For this review, take the finished solid that the model builds, in its own axes (mm). A direction names the side the tool comes from. Round coordinates to 2 decimals unless told otherwise and drop trailing zeros. Write each loop counter-clockwise with the first axis right and the second up, starting at its lowest first coordinate (ties: lowest second). Pieces come first, ordered by that corner, then holes. Notation, with made-up numbers: M 74,29 L 105,29 A22 cw 105,52 Z; hole C -6.5,45.25 d7. An arc over 180 degrees is marked long. One line per question, with ' | ' between items.
```python
from build123d import *

# Parameters (mm, degrees)
F1_DEPTH = 5
F2_W     = 3
F2_H     = 7
F3_DEPTH = 6


with BuildPart() as f1:
    # F0 (on Right) → F1 (new body, symmetric)
    with BuildSketch(Plane.YZ):
        with BuildLine():
            ThreePointArc((0, 4.6000001004), (-3.8076052812, 5.1521296368), (-7.460796192, 6.3591512489))
            ThreePointArc((-7.460796192, 6.3591512489), (-7.8828526102, 6.3468033059), (-8.1449647452, 6.0157726117))
            ThreePointArc((-8.1449647452, 6.0157726117), (-8.8517929002, 1.8362640656), (-9, -2.3999998996))
            Line((-9, -2.3999998996), (0, -2.3999998996))
            Line((0, -2.3999998996), (9, -2.3999998996))
            ThreePointArc((9, -2.3999998996), (8.8517929002, 1.8362640656), (8.1449647452, 6.0157726117))
            ThreePointArc((8.1449647452, 6.0157726117), (7.8828526102, 6.3468033059), (7.460796192, 6.3591512489))
            ThreePointArc((7.460796192, 6.3591512489), (3.8076052812, 5.1521296368), (0, 4.6000001004))
        make_face()
    extrude(amount=F1_DEPTH, both=True)

    # F2 (on face) → F3 (join)
    with BuildSketch(Plane(origin=(0, 0, -2.3999998996), x_dir=(1, 0, 0), z_dir=(0, 0, -1))):
        Rectangle(F2_W, F2_H)
    extrude(amount=F3_DEPTH)


solid = f1.part
```
Item 1: Take a section at C-C (y = -1.5). Write out the cut boundary in (x, z).
Results:
outline: M -5,-2.4 L -1.5,-2.4 L -1.5,-8.4 L 1.5,-8.4 L 1.5,-2.4 L 5,-2.4 L 5,4.74 L -5,4.74 Z
Item 2: Take a section at B-B (z = 5). Write out the cut boundary in (x, y), then the cut area to 3 significant figures.
Results:
outline: M -5,-8.37 L 5,-8.37 L 5,-3.11 L -5,-3.11 Z; M -5,3.11 L 5,3.11 L 5,8.37 L -5,8.37 Z | area: 105 mm2
Item 3: To check wall thickness, follow line 1 along Y through (x, z) = (3.5, -1.75); line 2 along X through (y, z) = (0.25, -2.75); line 3 along Y through (x, z) = (-1, -6). State the ranges of each line that lie inside material, in increasing order. Write a range as from..to.
Results:
line 1: -9.01..9.01 | line 2: -1.5..1.5 | line 3: -3.5..3.5
Item 4: Mouldability with a two-part tool opening along Y and no side actions: class faces 1 (the face through (0, -3.5, -5)), 2 (the face through (0, 0, -8.4)), 3 (the face through (0.07, -3.76, 5.14)) as +Y half, -Y half, draft (parallel to the pull), parting line (faces both ways), or undercut.
Results:
face 1: -Y half | face 2: draft | face 3: undercut
Item 5: Insertion check: pin 1 Ø2 at (x, y) = (-1.5, 6) entering from +Z; pin 2 Ø2.5 at (x, z) = (0.5, -5.5) entering from -Y; pin 3 Ø5 at (y, z) = (-0.5, -6) entering from -X; pin 4 Ø1 at (x, z) = (3.5, -5) entering from -Y. Each pin has a flat end and moves straight along its axis. Give the tip position at first contact, or say it passes through.
Results:
pin 1: z = 6.17 | pin 2: y = -3.5 | pin 3: x = -1.5 | pin 4: through
Item 6: Take a section at D-D (z = -4). Write out the cut boundary in (x, y).
Results:
outline: M -1.5,-3.5 L 1.5,-3.5 L 1.5,3.5 L -1.5,3.5 Z
Item 7: Machinability: for faces 4 (the face through (0.07, 3.86, 5.165)), 5 (the face through (0, 3.5, -5)), 6 (the face through (-1.5, 0, -5)), which of the approach directions +Z, -Z, +X, -X, +Y, -Y give a long, thin tool a straight path to every point of the face, cutting with its end or side? Answer none if there is none.
Results:
face 4: +Z, +X, -X | face 5: -Z, +X, -X, +Y | face 6: -Z, -X, +Y, -Y
Item 8: Take a section at A-A (x = 0). Write out the cut boundary in (y, z).
Results:
outline: M -9,-2.4 L -3.5,-2.4 L -3.5,-8.4 L 3.5,-8.4 L 3.5,-2.4 L 9,-2.4 A32 ccw 8.14,6.02 A0.5 ccw 7.46,6.36 A22 cw 0,4.6 A22 cw -7.46,6.36 A0.5 ccw -8.14,6.02 A32 ccw Z
